For this review, take the finished solid that the model builds, in its own axes (mm). Give positions to 0.01 mm unless a question says otherwise; leave off trailing zeros. Write each loop counter-clockwise with the first axis right and the second up, starting at its lowest first coordinate (ties: lowest second). Pieces come first, ordered by that corner, then holes. Notation, with made-up numbers: (20, -2.5) -> (47, -2.5) arc R25 ccw to (47, 22.5) -> close; hole circle Ø1 at (64.5, 72.5). An arc over 180 degrees is marked (long way). Return JSON: item names as keys, results as strings.
from build123d import *
from OCP.BRepFilletAPI import BRepFilletAPI_MakeChamfer

# Parameters (mm, degrees)
SKETCH1_R           = 8
BOSS_EXTRUDE1_DEPTH = 5
CUT_SWEEP1_PITCH    = 1.5
CHAMFER1_SIZE       = 0.3
CHAMFER1_SIZE2      = 0.139892297


with BuildPart() as part:
    # Sketch1 → Boss-Extrude1 (new body)
    with BuildSketch(Plane.XY):
        Polygon((10.165837862, 6.376185425), (-0.439019626, 11.991966551), (-10.604857488, 5.615781126), (-10.165837862, -6.376185425), (0.439019626, -11.991966551), (10.604857488, -5.615781126), align=None)
        Circle(SKETCH1_R, mode=Mode.SUBTRACT)
    extrude(amount=BOSS_EXTRUDE1_DEPTH)

    # Cut-Sweep1: arcs per turn and ends read off the stored shape
    # Cut-Sweep1: the profile of Sketch3 screwed along a right-hand helix through 5 turns, 8 arcs to a turn; built about Z, then put on its axis
    cut_sweep1_z = Axis((0, 0, 0), (0, 0, 1))
    cut_sweep1_corners = [(7.851099618, 5.3441e-05, -1.046060596), (7.851099618, 5.3441e-05, -2.046060596), (8.387226348, 5.709e-05, -1.796060596), (8.387226348, 5.709e-05, -1.296060596)]
    with BuildLine(mode=Mode.PRIVATE) as cut_sweep1_profile:
        Line(cut_sweep1_corners[0], cut_sweep1_corners[1])
        Line(cut_sweep1_corners[1], cut_sweep1_corners[2])
        Line(cut_sweep1_corners[2], cut_sweep1_corners[3])
        Line(cut_sweep1_corners[3], cut_sweep1_corners[0])
    cut_sweep1_cap = Face(cut_sweep1_profile.wire())
    cut_sweep1_turn_angles = [0, 22.5, 45, 67.5, 90, 112.5, 135, 157.5, 180, 202.5, 225, 247.5, 270, 292.5, 315, 337.5, 360]
    cut_sweep1_turn_weights = [1, 0.9238795325112867, 1, 0.9238795325112867, 1, 0.9238795325112867, 1, 0.9238795325112867, 1, 0.9238795325112867, 1, 0.9238795325112867, 1, 0.9238795325112867, 1, 0.9238795325112867, 1]
    cut_sweep1_turn_rails = [Edge.make_bspline([Vector(p[0], p[1], 0).rotate(cut_sweep1_z, cut_sweep1_turn_angles[k]) / cut_sweep1_turn_weights[k] + Vector(0, 0, p[2] + CUT_SWEEP1_PITCH * cut_sweep1_turn_angles[k] / 360) for k in range(17)], [0, 0, 0, 1, 1, 2, 2, 3, 3, 4, 4, 5, 5, 6, 6, 7, 7, 8, 8, 8], 2, cut_sweep1_turn_weights) for p in cut_sweep1_corners]
    cut_sweep1_turn_sides = [Face.make_surface_from_curves(cut_sweep1_turn_rails[p[0]], cut_sweep1_turn_rails[p[1]]) for p in [(0, 1), (1, 2), (2, 3), (3, 0)]]
    cut_sweep1 = Plane(origin=(0, 0, 5), x_dir=(1, 0, 0), z_dir=(0, 0, -1)) * Solid(Shell([*[p.moved(Location((0, 0, CUT_SWEEP1_PITCH * i))) for i in range(5) for p in cut_sweep1_turn_sides], cut_sweep1_cap, cut_sweep1_cap.rotate(cut_sweep1_z, 1800).moved(Location((0, 0, CUT_SWEEP1_PITCH * 1800 / 360)))]))
    add(cut_sweep1, mode=Mode.SUBTRACT)

    # Chamfer1: one chamfer whose edges measure the first distance from different faces: ONE call of the kernel's chamfer builder (chamfer() names one face for all edges)
    chamfer1_edges_1 = [part.edges().sort_by_distance(p)[0] for p in [
        (-5.521938557, 8.803873839, 5),
    ]]
    chamfer1_side_1 = [part.faces().sort_by_distance(p)[0] for p in [
        (-5.521938557, 8.803873839, 2.5),
    ]]
    chamfer1_edges_2 = [part.edges().sort_by_distance(p)[0] for p in [
        (-10.385347675, -0.380202149, 5),
    ]]
    chamfer1_side_2 = [part.faces().sort_by_distance(p)[0] for p in [
        (-10.385347675, -0.380202149, 2.5),
    ]]
    chamfer1_edges_3 = [part.edges().sort_by_distance(p)[0] for p in [
        (-4.863409118, -9.184075988, 5),
    ]]
    chamfer1_side_3 = [part.faces().sort_by_distance(p)[0] for p in [
        (-4.863409118, -9.184075988, 2.5),
    ]]
    chamfer1_edges_4 = [part.edges().sort_by_distance(p)[0] for p in [
        (5.521938557, -8.803873839, 5),
    ]]
    chamfer1_side_4 = [part.faces().sort_by_distance(p)[0] for p in [
        (5.521938557, -8.803873839, 2.5),
    ]]
    chamfer1_edges_5 = [part.edges().sort_by_distance(p)[0] for p in [
        (10.385347675, 0.380202149, 5),
    ]]
    chamfer1_side_5 = [part.faces().sort_by_distance(p)[0] for p in [
        (10.385347675, 0.380202149, 2.5),
    ]]
    chamfer1_edges_6 = [part.edges().sort_by_distance(p)[0] for p in [
        (5.521938557, -8.803873839, 0),
        (-4.863409118, -9.184075988, 0),
        (-10.385347675, -0.380202149, 0),
        (-5.521938557, 8.803873839, 0),
        (4.863409118, 9.184075988, 0),
        (10.385347675, 0.380202149, 0),
    ]]
    chamfer1_side_6 = [part.faces().sort_by_distance(p)[0] for p in [
        (4.713575925, 8.901130549, 0),
    ]]
    chamfer1_edges_7 = [part.edges().sort_by_distance(p)[0] for p in [
        (4.863409118, 9.184075988, 5),
    ]]
    chamfer1_side_7 = [part.faces().sort_by_distance(p)[0] for p in [
        (4.863409118, 9.184075988, 2.5),
    ]]
    chamfer1 = BRepFilletAPI_MakeChamfer(part.part.solid().wrapped)
    for e in chamfer1_edges_1:
        chamfer1.Add(CHAMFER1_SIZE, CHAMFER1_SIZE2, e.wrapped, chamfer1_side_1[0].wrapped)  # the first distance lies on this face
    for e in chamfer1_edges_2:
        chamfer1.Add(CHAMFER1_SIZE, CHAMFER1_SIZE2, e.wrapped, chamfer1_side_2[0].wrapped)  # the first distance lies on this face
    for e in chamfer1_edges_3:
        chamfer1.Add(CHAMFER1_SIZE, CHAMFER1_SIZE2, e.wrapped, chamfer1_side_3[0].wrapped)  # the first distance lies on this face
    for e in chamfer1_edges_4:
        chamfer1.Add(CHAMFER1_SIZE, CHAMFER1_SIZE2, e.wrapped, chamfer1_side_4[0].wrapped)  # the first distance lies on this face
    for e in chamfer1_edges_5:
        chamfer1.Add(CHAMFER1_SIZE, CHAMFER1_SIZE2, e.wrapped, chamfer1_side_5[0].wrapped)  # the first distance lies on this face
    for e in chamfer1_edges_6:
        chamfer1.Add(CHAMFER1_SIZE, CHAMFER1_SIZE2, e.wrapped, chamfer1_side_6[0].wrapped)  # the first distance lies on this face
    for e in chamfer1_edges_7:
        chamfer1.Add(CHAMFER1_SIZE, CHAMFER1_SIZE2, e.wrapped, chamfer1_side_7[0].wrapped)  # the first distance lies on this face
    add(Compound.cast(chamfer1.Shape()), mode=Mode.REPLACE)


solid = part.part
1. Add section A-A, the plane y = -9.25. State the section outline as (x, z) points, plus the area to 3 significant figures.
Results found:
{"outline": "(-4.74, 0.14) -> (-4.1, 0) -> (4.25, 0) -> (4.81, 0.14) -> (4.81, 4.7) -> (4.55, 5) -> (-4.44, 5) -> (-4.74, 4.7) -> close", "area": "47.6 mm²"}
2. To check wall thickness, follow probe 1 along X at (y, z) = (0, 3.6); probe 2 along X at (y, z) = (-4.5, 3); probe 3 along Y at (x, z) = (0.75, 3). State the ranges of each line that lie inside material, in increasing order.
Results found:
{"probe 1": "x = -10.4 to -8, 8.39 to 10.4", "probe 2": "x = -10.23 to -7.08, 6.68 to 10.56", "probe 3": "y = -11.8 to -8.35, 7.96 to 11.36"}
3. For pin 1 (2 mm diameter, centred on y = 3.5, z = 1.5, fed in from -X); pin 2 (9.5 mm diameter, centred on x = 0, y = 0, fed in from +Z); pin 3 (1.5 mm diameter, centred on y = -3.5, z = 3, fed in from +X); pin 4 (10 mm diameter, centred on x = 3, y = -2, fed in from +Z), all flat-tipped, find the tip position at first contact; note any pin that passes through.
Results found:
{"pin 1": "stops at x = -10.56", "pin 2": "passes through", "pin 3": "stops at x = 10.55", "pin 4": "stops at z = 5"}
